Could you check a few things on this model? Use its own coordinates, in mm. Face numbers are marked on the shaded views. Round coordinates to 2 decimals unless told otherwise and drop trailing zeros. Order: outer loops, then holes, each group sorted by start corner. A loop starts at its lowest first (then second) coordinate and runs counter-clockwise, first axis right, second up. Notation, with made-up numbers: M -8,78 L 2,78 A15 ccw 2,101 Z; hole C 16.25,12 d11. An arc over 180 degrees is marked long. Write each question's results on one line, items separated by ' | '. Start each with the question number.
1. Suppose I cut it at A-A on y = 8. Write out the boundary of the cut face in (x, z).
2. We'd pull the mould along Y, two halves only. Please class the marked faces 1, 2 and 3: released by +Y, released by -Y, zero draft, split by the parting line, or undercut.
3. Please list where these lines run through material, in increasing order: L1, parallel to Z at x = 3, y = -9; L2, parallel to Y at x = 8.5, z = 0; L3, parallel to Y at x = 4, z = 2.
4. Suppose I cut it at B-B on x = 5. Give the number of separate pieces and of enclosed holes in the cut face, and give its area (3 significant figures).
5. I'm going to push flat-ended pins straight in: pin 1 (6.5 mm diameter, centred on y = 15.81, z = 20.65, fed in from -X); pin 2 (4.5 mm diameter, centred on y = -44.94, z = -4.1, fed in from +X); pin 3 (6.5 mm diameter, centred on y = -114.94, z = -4.1, fed in from +X). Where does each tip first touch, or does it pass through?
6. Suppose I cut it at C-C on z = 8. Write out the boundary of the cut face in (x, y), and give its area (3 significant figures).
from build123d import *

# Parameters (mm, degrees)
SKETCH_1_W          = 60
SKETCH_1_H          = 180
EXTRUDE_1_DEPTH     = 10
SKETCH_2_R          = 14.5
CUT_EXTRUDE_1_DEPTH = 30
SKETCH_3_R          = 2
CUT_EXTRUDE_2_DEPTH = 10
CHAMFER_2_SIZE      = 2
SKETCH_4_R          = 2
CUT_EXTRUDE_3_DEPTH = 15
CHAMFER_3_SIZE      = 2.9
CHAMFER_4_SIZE      = 10
SKETCH_5_R          = 1.65
CUT_EXTRUDE_4_DEPTH = 15


with BuildPart() as part:
    # Эскиз1 → Бобышка-Вытянуть1 (new body)
    with BuildSketch(Plane(origin=(0, 0, 0), x_dir=(0, 0, -1), z_dir=(1, 0, 0))):
        with Locations((4.096360158, -39.937525072)):
            Rectangle(SKETCH_1_W, SKETCH_1_H)
    extrude(amount=EXTRUDE_1_DEPTH)

    # Эскиз2 → Вырез-Вытянуть1 (cut)
    with BuildSketch(Plane.ZY):
        with Locations((-4.096360158, 1.062474928)):
            Circle(SKETCH_2_R)
    extrude(amount=-CUT_EXTRUDE_1_DEPTH, mode=Mode.SUBTRACT)

    # Эскиз3 → Вырез-Вытянуть2 (cut)
    with BuildSketch(Plane.ZY):
        with Locations((-28.8450975, 15.811212269)):
            Circle(SKETCH_3_R)
        with Locations((-28.8450975, -33.686262414)):
            Circle(SKETCH_3_R)
        with Locations((20.652377183, 15.811212269)):
            Circle(SKETCH_3_R)
        with Locations((20.652377183, -33.686262414)):
            Circle(SKETCH_3_R)
    extrude(amount=-CUT_EXTRUDE_2_DEPTH, mode=Mode.SUBTRACT)

    # Фаска2
    chamfer_2_edges = [part.edges().sort_by_distance(p)[0] for p in [
        (0, 15.811212269, -30.8450975),
        (0, -33.686262414, -30.8450975),
        (0, 15.811212269, 18.652377183),
        (0, -33.686262414, 18.652377183),
    ]]
    chamfer(chamfer_2_edges, length=CHAMFER_2_SIZE)

    # Эскиз4 → Вырез-Вытянуть3 (cut)
    with BuildSketch(Plane(origin=(10, 0, 0), x_dir=(0, 0, -1), z_dir=(1, 0, 0))):
        with Locations((4.096360158, -114.937525072)):
            Circle(SKETCH_4_R)
        with Locations((4.096360158, -44.937525072)):
            Circle(SKETCH_4_R)
        with Locations((4.096360158, 35.062474928)):
            Circle(SKETCH_4_R)
    extrude(amount=-CUT_EXTRUDE_3_DEPTH, mode=Mode.SUBTRACT)

    # Фаска3
    chamfer_3_edges = [part.edges().sort_by_distance(p)[0] for p in [
        (10, -114.937525072, -2.096360158),
        (10, -44.937525072, -2.096360158),
        (10, 35.062474928, -2.096360158),
    ]]
    chamfer(chamfer_3_edges, length=CHAMFER_3_SIZE)

    # Фаска4
    chamfer_4_edges = [part.edges().sort_by_distance(p)[0] for p in [
        (5, 50.062474928, 25.903639842),
        (5, 50.062474928, -34.096360158),
    ]]
    chamfer(chamfer_4_edges, length=CHAMFER_4_SIZE)

    # Эскиз5 → Вырез-Вытянуть4 (cut)
    with BuildSketch(Plane.XZ.offset(129.937525072)):
        with Locations(Location((5, 19.903639842, 0), (0, 0, 270))):
            Circle(SKETCH_5_R)
        with Locations(Location((5, -28.096360158, 0), (0, 0, 270))):
            Circle(SKETCH_5_R)
    extrude(amount=-CUT_EXTRUDE_4_DEPTH, mode=Mode.SUBTRACT)


solid = part.part
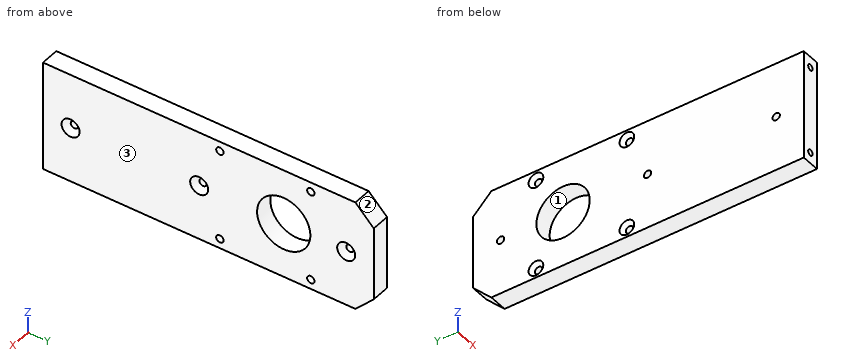
Filled sheet:
1) outline: M 0,-34.1 L 10,-34.1 L 10,-16.83 L 0,-16.83 Z; M 0,8.64 L 10,8.64 L 10,25.9 L 0,25.9 Z
2) face 1: undercut | face 2: released by +Y | face 3: zero draft
3) L1: z = -34.1 to -14.54, 6.34 to 25.9 | L2: y = -129.94 to -12.85, 14.97 to 50.06 | L3: y = -129.94 to -12.09, 14.22 to 50.06
4) separate pieces: 1 | enclosed holes: 8 | area: 9,850 mm^2
5) pin 1: stops at x = 0.75 | pin 2: stops at x = 7.35 | pin 3: stops at x = 8.35
6) outline: M 0,-129.94 L 10,-129.94 L 10,-6.93 L 0,-6.93 Z; M 0,9.06 L 10,9.06 L 10,50.06 L 0,50.06 Z | area: 1,640 mm^2
